Here's the drawing with two shaded views (mm, measured from the low corner). I have some questions. Round coordinates to 2 decimals unless told otherwise and drop trailing zeros. Loops run counter-clockwise (first coordinate to the right, second up) from the corner with the lowest first, then second, coordinate; pieces in that order, holes last.
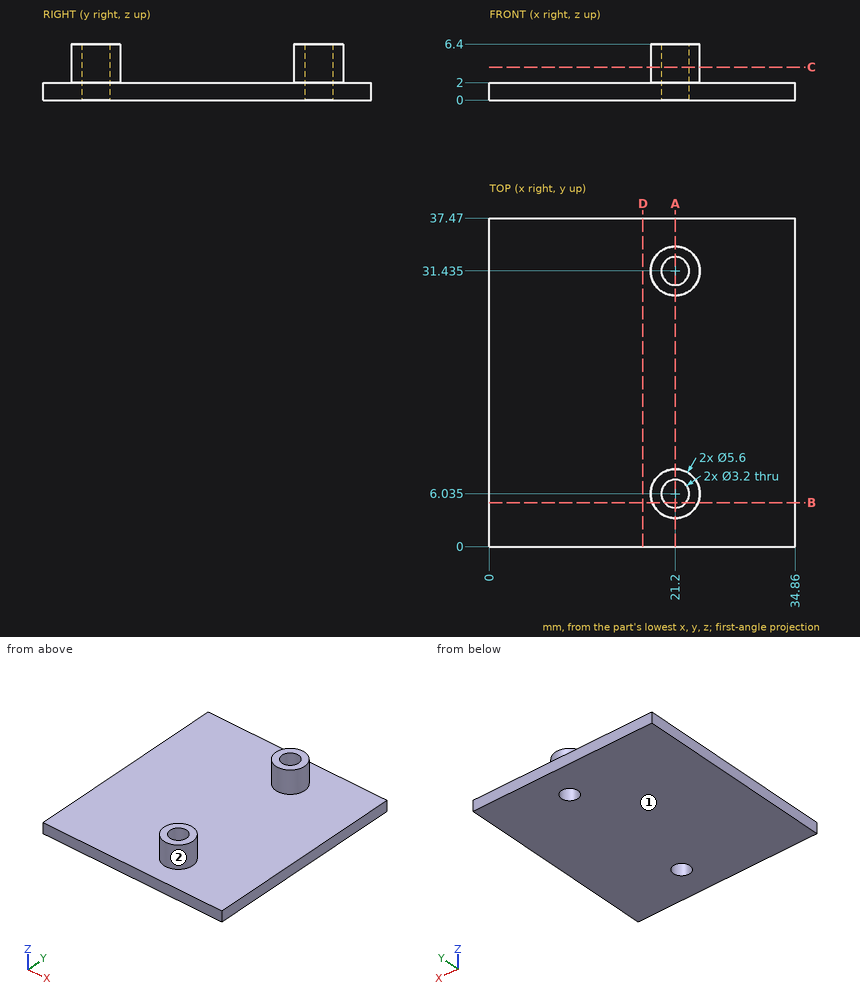
Item 1: If I drill on line 1 along Y through (x, z) = (21.2, 1.5) (3 decimals); line 2 along Y through (x, z) = (21.2, 3) (3 decimals); line 3 along Z through (x, y) = (29, 34.5), over which ranges is the centre line in solid material (lowest first)?
Results list:
line 1: y = 0 to 4.435, 7.635 to 29.835, 33.035 to 37.47
line 2: y = 3.235 to 4.435, 7.635 to 8.835, 28.635 to 29.835, 33.035 to 34.235
line 3: z = 0 to 2
Item 2: If we section it at A-A, the plane x = 21.2: Please give me the cut outline in (y, z) (3 decimals), then the cut area to 3 significant figures.
Results list:
outline: (0, 0) - (4.435, 0) - (4.435, 6.4) - (3.235, 6.4) - (3.235, 2) - (0, 2) - close; (7.635, 0) - (29.835, 0) - (29.835, 6.4) - (28.635, 6.4) - (28.635, 2) - (8.835, 2) - (8.835, 6.4) - (7.635, 6.4) - close; (33.035, 0) - (37.47, 0) - (37.47, 2) - (34.235, 2) - (34.235, 6.4) - (33.035, 6.4) - close
area: 83.3 mm2
Item 3: If we section it at B-B, the plane y = 5: Please give me the cut outline in (x, z), then the cut area to 3 significant figures.
Results list:
outline: (0, 0) - (19.98, 0) - (19.98, 6.4) - (18.6, 6.4) - (18.6, 2) - (0, 2) - close; (22.42, 0) - (34.86, 0) - (34.86, 2) - (23.8, 2) - (23.8, 6.4) - (22.42, 6.4) - close
area: 77.0 mm2
Item 4: Will these pins go through, and if not, where does the flat tip stop? pin 1 (1 mm diameter, centred on x = 13.5, y = 16.5, fed in from +Z); pin 2 (3 mm diameter, centred on y = 9, z = 4.5, fed in from +X).
Results list:
pin 1: stops at z = 2
pin 2: stops at x = 23.59
Item 5: If we section it at D-D, the plane x = 17.5: Please give me the cut outline in (y, z).
Results list:
outline: (0, 0) - (37.47, 0) - (37.47, 2) - (0, 2) - close
Item 6: We'd pull the mould along Y, two halves only. Please class the marked faces 1 and 2: released by +Y, released by -Y, zero draft, split by the parting line, or undercut.
Results list:
face 1: zero draft
face 2: undercut
Item 7: If we section it at C-C, the plane z = 3.75: Please give me the cut outline in (x, y) (3 decimals), then the cut area to 3 significant figures.
Results list:
outline: circle Ø5.6 at (21.2, 6.035); circle Ø5.6 at (21.2, 31.435); hole circle Ø3.2 at (21.2, 6.035); hole circle Ø3.2 at (21.2, 31.435)
area: 33.2 mm2
